from build123d import *

# Parameters (mm, degrees)
BOSS_EXTRUDE1_DEPTH = 134.9375
SKETCH4_W           = 25.4
SKETCH4_H           = 19.05
CUT_EXTRUDE1_DEPTH  = 6.35
SKETCH5_R           = 2.921
CUT_EXTRUDE2_DEPTH  = 25.4
CUT_EXTRUDE3_DEPTH  = 38.1
CUT_EXTRUDE3_TAPER  = -1


with BuildPart() as part:
    # Sketch3 → Boss-Extrude1 (new body)
    with BuildSketch(Plane(origin=(0, 0, 0), x_dir=(0, 0, -1), z_dir=(1, 0, 0))):
        with BuildLine():
            Line((0, 0), (95.25, 0))
            Line((95.25, 0), (95.25, 44.45))
            ThreePointArc((95.25, 44.45), (49.555547135, 18.088113282), (0, 0))
        make_face()
    extrude(amount=BOSS_EXTRUDE1_DEPTH)

    # Sketch4 → Cut-Extrude1 (cut)
    with BuildSketch(Plane.ZY):
        with Locations((-82.55, 17.145)):
            Rectangle(SKETCH4_W, SKETCH4_H)
    extrude(amount=-CUT_EXTRUDE1_DEPTH, mode=Mode.SUBTRACT)

    # Sketch5 → Cut-Extrude2 (cut)
    with BuildSketch(Plane.ZY.offset(-6.35)):
        with Locations((-82.55, 17.145)):
            Circle(SKETCH5_R)
    extrude(amount=-CUT_EXTRUDE2_DEPTH, mode=Mode.SUBTRACT)

    # Sketch6 → Cut-Extrude3 (cut)
    with BuildSketch(Plane.XZ):
        Polygon((134.9375, -82.55), (134.9375, -72.39), (127.014719298, -70.993), (127.014719298, -83.947), align=None)
        Polygon((134.9375, -62.822666667), (134.9375, -52.662666667), (127.014719298, -51.265666667), (127.014719298, -64.219666667), align=None)
        Polygon((134.9375, -43.095333333), (134.9375, -32.935333333), (127.014719298, -31.538333333), (127.014719298, -44.492333333), align=None)
        Polygon((134.9375, -23.368), (134.9375, -13.208), (127.014719298, -11.811), (127.014719298, -24.765), align=None)
    extrude(amount=-CUT_EXTRUDE3_DEPTH, taper=CUT_EXTRUDE3_TAPER, mode=Mode.SUBTRACT)


solid = part.part
Design review of the part built by this model. Coordinates are the model's own, in mm. A direction names the side the tool comes from. Round coordinates to 2 decimals unless told otherwise and drop trailing zeros. Write each loop counter-clockwise with the first axis right and the second up, starting at its lowest first coordinate (ties: lowest second). Pieces come first, ordered by that corner, then holes. Notation, with made-up numbers: (-17, 70) - (8, 70) arc R15 cw to (8, 94) - close; hole circle Ø3 at (-11, 50.25). An arc over 180 degrees is marked (long way). Return JSON: item names as keys, results as strings. Group by question number.
Item 1: For probe 1 along Y at (x, z) = (25.25, -82.55); probe 2 along Z at (x, y) = (11.5, 19); probe 3 along X at (y, z) = (10, -70), list the stretches that pass through material, from the lowest coordinate up. Write a range as [from, to].
Item 2: Insertion check: P1, Ø1.5, axis at x = 67, z = -71, coming from the +Y side; P2, Ø5, axis at x = 118, y = 22, coming from the +Z side; P3, Ø1.9, axis at x = 4.5, y = 14, coming from the -Z side. Each pin has a flat end and moves straight along its axis. Give the tip position at first contact, or say it passes through.
Item 3: Machinability: for faces 1 (the face through (31.75, 17, -83)), 2 (the face through (134.938, 1, -9)), 3 (the face through (6.35, 17, -86)), which of the approach directions +Z, -Z, +X, -X, +Y, -Y give a long, thin tool a straight path to every point of the face, cutting with its end or side? Answer none if there is none.
Item 4: We need section A-A on x = 89.5. Write out the cut boundary in (y, z), and give its area (3 significant figures).
Item 5: The part is to be moulded in two halves that separate along Z. For faces 4 (the face through (67, 22, -95.25)), 5 (the face through (18.872, 18.022, -79.764)), 6 (the face through (3, 7.62, -83)), say which applies: pulls with the +Z half, pulls with the -Z half, needs draft (parallel to the pull), parting line crosses it, or undercut.
Model answer:
{
 "1": {"probe 1": "y = [0, 14.22], [20.07, 36.04]", "probe 2": "z = [-95.25, -84.81], [-80.29, -51.49]", "probe 3": "x = [6.35, 134.94]"},
 "2": {"P1": "stops at y = 29.58", "P2": "stops at z = -52.54", "P3": "stops at z = -69.85"},
 "3": {"face 1": "-X", "face 2": "+Z, -Z, +X, +Y, -Y", "face 3": "-Z, -X"},
 "4": {"outline": "(0, -95.25) - (44.45, -95.25) arc R304.8 cw to (0, 0) - close", "area": "1,800 mm²"},
 "5": {"face 4": "pulls with the -Z half", "face 5": "undercut", "face 6": "needs draft"}
}
